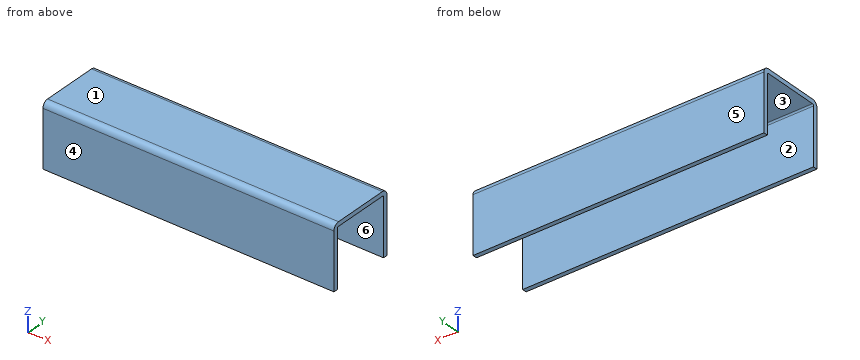
from build123d import *

# Parameters (mm, degrees)
BOSS_EXTRUDE1_DEPTH    = 100
CONVERT_SOLID1_START   = -100
CONVERT_SOLID1_DEPTH   = 200
CONVERT_SOLID1_2_DEPTH = 200


# Read off the part's stored shape, not the designer's step: Convert-Solid1
with BuildPart() as part:
    # Sketch1 → Boss-Extrude1 (new, symmetric)
    with BuildSketch(Plane(origin=(0, 0, 0), x_dir=(0, 0, -1), z_dir=(1, 0, 0))):
        Polygon((0, 0), (0, -40.5), (40, -40.5), (40, -43.5), (-3, -43.5), (-3, 3), (40, 3), (40, 0), align=None)
    extrude(amount=BOSS_EXTRUDE1_DEPTH, both=True)

    # Convert-Solid1 outline → Convert-Solid1 (cut)
    with BuildSketch(Plane.YZ.offset(CONVERT_SOLID1_START)):
        with BuildLine():
            Line((3, 3), (-1, 3))
            ThreePointArc((-1, 3), (1.828427125, 1.828427125), (3, -1))
            Line((3, -1), (3, 3))
        make_face()
        with BuildLine():
            ThreePointArc((-43.5, -1), (-42.328427125, 1.828427125), (-39.5, 3))
            Line((-39.5, 3), (-43.5, 3))
            Line((-43.5, 3), (-43.5, -1))
        make_face()
    extrude(amount=CONVERT_SOLID1_DEPTH, mode=Mode.SUBTRACT)

    # Convert-Solid1 2 outline → Convert-Solid1 2 (add)
    with BuildSketch(Plane.YZ.offset(CONVERT_SOLID1_START)):
        with BuildLine():
            Line((0, 0), (-1, 0))
            ThreePointArc((-1, 0), (-0.292893219, -0.292893219), (0, -1))
            Line((0, -1), (0, 0))
        make_face()
        with BuildLine():
            ThreePointArc((-40.5, -1), (-40.207106781, -0.292893219), (-39.5, 0))
            Line((-39.5, 0), (-40.5, 0))
            Line((-40.5, 0), (-40.5, -1))
        make_face()
    extrude(amount=CONVERT_SOLID1_2_DEPTH)


solid = part.part
Source: CAD feature listing. Evaluate the final solid. Frame: model axes, mm. Face numbers are marked on the shaded views. A direction names the side the tool comes from. Coordinates: 2 decimals unless noted, no trailing zeros. Loops run counter-clockwise (first coordinate to the right, second up) from the corner with the lowest first, then second, coordinate; pieces in that order, holes last. Notation, with made-up numbers: M 14,42 L 20,42 A30 ccw 20,81 Z; hole C -38.5,61 d8. An arc over 180 degrees is marked long. Answer in a Markdown table with one row per item.
Q1. Draft query along Y for the marked faces 3, 4, 5 and 6. Return one class per face: pulls with the +Y half, pulls with the -Y half, needs draft (parallel to the pull), parting line crosses it, or undercut.
Answers below:
| item | result |
|---|---|
| face 3 | undercut |
| face 4 | pulls with the -Y half |
| face 5 | pulls with the +Y half |
| face 6 | undercut |
Q2. First-contact query: pin 1 (6 mm diameter, centred on y = -3.5, z = -21, fed in from +X); pin 2 (12 mm diameter, centred on x = -39.5, y = -12.5, fed in from -Z). Flat tips, straight axial feed; report the tip coordinate or a pass-through.
Answers below:
| item | result |
|---|---|
| pin 1 | passes through |
| pin 2 | stops at z = 0 |
Q3. Section C-C on y = -29. Return the cut outline in (x, z).
Answers below:
| item | result |
|---|---|
| outline | M -100,0 L 100,0 L 100,3 L -100,3 Z |
Q4. Ray query, probe 1 along Y at (x, z) = (-7.5, -11); probe 2 along Z at (x, y) = (-39.5, -21); probe 3 along Z at (x, y) = (86.5, -40). Return the intervals inside material, ascending. Write a range as from..to.
Answers below:
| item | result |
|---|---|
| probe 1 | y = -43.5..-40.5, 0..3 |
| probe 2 | z = 0..3 |
| probe 3 | z = -0.13..2.97 |
Q5. Set-up query: the marked faces 1 and 2. Return all of +Z, -Z, +X, -X, +Y, -Y with unobstructed straight access to the full face (end or side cutting, diameter ignored); none if empty.
Answers below:
| item | result |
|---|---|
| face 1 | +Z, +X, -X, +Y, -Y |
| face 2 | -Z, +X, -X |
Q6. Section B-B on x = 67.5. Return the cut outline in (y, z).
Answers below:
| item | result |
|---|---|
| outline | M -43.5,-40 L -40.5,-40 L -40.5,-1 A1 cw -39.5,0 L -1,0 A1 cw 0,-1 L 0,-40 L 3,-40 L 3,-1 A4 ccw -1,3 L -39.5,3 A4 ccw -43.5,-1 Z |
Q7. Section A-A on z = -31.5. Return the cut outline in (x, y).
Answers below:
| item | result |
|---|---|
| outline | M -100,-43.5 L 100,-43.5 L 100,-40.5 L -100,-40.5 Z; M -100,0 L 100,0 L 100,3 L -100,3 Z |
